Input: part model. Units: mm. Frame: model coordinates. Give positions to 0.01 mm unless a question says otherwise; leave off trailing zeros. Write each loop counter-clockwise with the first axis right and the second up, starting at its lowest first coordinate (ties: lowest second). Pieces come first, ordered by that corner, then holes. Notation, with made-up numbers: (-4.5, -4) - (7.5, -4) arc R15 cw to (7.5, 23) - close; hole circle Ø1 at (39, 61). An arc over 180 degrees is marked (long way). Use a Markdown table: item, result. Add a question column.
1. Section query A-A, the plane y = 24. Return loops of the section in (x, z), plus the area to 3 significant figures.
2. Material intervals for probe 1 along Y at (x, z) = (82, 1.5); probe 2 along Y at (x, z) = (57.5, 1.5); probe 3 along Y at (x, z) = (76.5, 2.25), sorted ascending.
3. Section query C-C, the plane x = 135.5. Return loops of the section in (y, z), plus the area to 3 significant figures.
4. Section query B-B, the plane x = 54. Return loops of the section in (y, z), plus the area to 3 significant figures.
5. Pin query (flat end, axial travel): pin 1 (0.9 mm diameter, centred on x = 24.5, y = 2, fed in from +Z); pin 2 (1.3 mm diameter, centred on x = 52.5, y = 14, fed in from +Z); pin 3 (2 mm diameter, centred on y = 10, z = 0, fed in from -X); pin 4 (10 mm diameter, centred on x = 81.5, y = 11.5, fed in from -Z). Return the tip coordinate at first contact, or that it passes through.
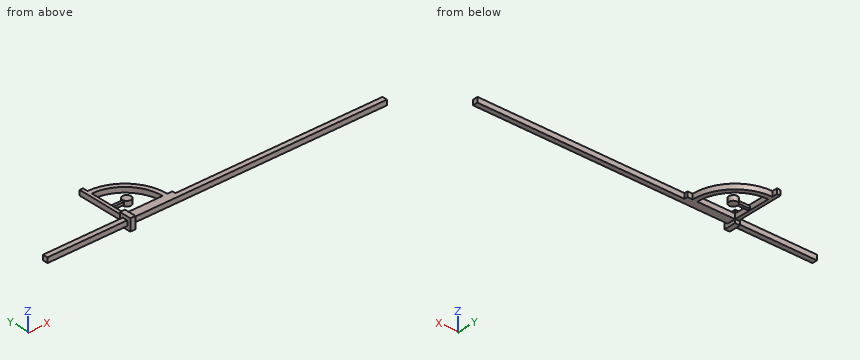
Autodesk Inventor part; units mm, degrees
ref_plane "YZ Plane" through (0, 0, 0) normal (1, 0, 0) x (0, 1, 0)
ref_plane "XZ Plane" through (0, 0, 0) normal (0, 1, 0) x (-1, 0, 0)
ref_plane "XY Plane" through (0, 0, 0) normal (0, 0, 1) x (1, 0, 0)
sketch "Skizze4" plane through (0, 0, 0) normal (0, 0, 1) x (1, 0, 0)
  line L0 (0, 0) -> (200, 0)
  line L1 (200, 0) -> (200, 3)
  line L2 (200, 3) -> (0, 3)
  line L3 (0, 3) -> (0, 0)
  dimension "d12" = 200
  dimension "d13" = 3
extrude "Extrusion4" add sketch "Skizze4" along normal blind 3
sketch "Skizze5" plane through (0, 0, 3) normal (0, 0, 1) x (1, 0, 0)
  line L0 (47, 5) -> (50, 5)
  line L1 (50, 5) -> (50, -2)
  line L2 (50, -2) -> (47, -2)
  line L3 (47, -2) -> (47, 5)
  line L4 (200, 0) -> (200, 3)
  line L5 (0, 3) -> (0, 0)
  line L6 (200, 3) -> (0, 3)
  line L7 (0, 0) -> (200, 0)
  dimension "d16" = 150
  dimension "d17" = 47
  dimension "d18" = 2
  dimension "d19" = 2
extrude "Extrusion5" add sketch "Skizze5" along normal blind 2 and the other way blind 5 contours L0 L1 L6 L3 | L6 L1 L7 L3 | L7 L1 L2 L3
sketch "Skizze6" plane through (0, 0, -2) normal (0, 0, -1) x (-1, 0, 0)
  point P0 (0, 0)
sketch "Skizze7" plane through (0, 0, 0) normal (0, 0, -1) x (-1, 0, 0)
  line L0 (-200, 3) -> (-50, 3)
  line L1 (-78, 3) -> (-50, 3)
  line L2 (-50, 3) -> (-50, 5)
  line L3 (-50, 5) -> (-78, 5)
  line L4 (-78, 5) -> (-78, 3)
  line L5 (-50, 5) -> (-48, 5)
  line L6 (-48, 5) -> (-48, 33)
  line L7 (-48, 33) -> (-50, 33)
  line L8 (-50, 33) -> (-50, 5)
  line L9 (-50, -2) -> (-50, 5)
  arc A0 (-50, 30) -> (-75, 5) centre (-50, 5) ccw
  arc A1 (-50, 27.2) -> (-72.2, 5) centre (-50, 5) ccw
  line L10 (-50, 5) -> (-59.1924, 14.1924)
  line L11 (-50, 5) -> (-37, 5) construction
  circle A2 centre (-59.1924, 14.1924) radius 2.5
  line L12 (-59.1924, 14.1924) -> (-50, 14.1924)
  line L13 (-59.1924, 14.1924) -> (-50, 14.1924)
  line L14 (-50, 14.1924) -> (-50, 13.3924)
  line L15 (-50, 13.3924) -> (-59.1924, 13.3924)
  line L16 (-59.1924, 13.3924) -> (-59.1924, 14.1924)
  line L17 (-50, 14.1924) -> (-59.1924, 14.1924)
  line L18 (-59.1924, 14.1924) -> (-59.1924, 14.9924)
  line L19 (-59.1924, 14.9924) -> (-50, 14.9924)
  line L20 (-50, 14.9924) -> (-50, 14.1924)
  line L21 (-50, 30) -> (-50, 27.2)
  line L22 (-75, 5) -> (-72.2, 5)
  point P0 (0, 0)
  dimension "d24" = 2
  dimension "d25" = 2
  dimension "d26" = 50
  dimension "d27" = 2.8
  dimension "d28" = 13
  dimension "d29" = 135
  dimension "d30" = 5
  dimension "d31" = 0.8
  dimension "d32" = 0.8
  dimension "d33" = 28
  dimension "d34" = 28
extrude "Extrusion6" add sketch "Skizze7" against normal blind 3 contours L4 L3 L2 L0 | L8 L7 L6 L5 | A0 L8 A1 L3 | L15 A2 L12 L8 | A2 L19 L18 L16 L15 L10 | L10 L15 A2 | L12 A2 L19 L8 | L15 L10 L12 A2 | L15 L16 L10 | A2 L12 L18 L19
sketch "Skizze8" plane through (0, 0, 0) normal (0, 0, -1) x (-1, 0, 0)
  arc A0 (-56.8238, 14.9924) -> (-56.8238, 13.3924) centre (-59.1924, 14.1924) ccw
  circle A1 centre (-59.1924, 14.1924) radius 2.5
  line L0 (-56.8238, 13.3924) -> (-50, 13.3924)
  line L1 (-56.8238, 13.3924) -> (-50, 13.3924)
  line L2 (-50, 13.3924) -> (-50, 14.9924)
  line L3 (-56.8238, 14.9924) -> (-50, 14.9924)
  line L4 (-50, 14.9924) -> (-56.8238, 14.9924)
  point P0 (0, 0)
extrude "Extrusion7" cut sketch "Skizze8" against normal blind 0.75 contours L3 L2 L0 A1
sketch "Skizze9" plane through (0, 0, 3) normal (0, 0, 1) x (1, 0, 0)
  arc A0 (56.8238, 13.3924) -> (56.8238, 14.9924) centre (59.1924, 14.1924) ccw
  circle A1 centre (59.1924, 14.1924) radius 2.5
  line L0 (50, 14.9924) -> (50, 27.2)
  line L1 (56.8238, 14.9924) -> (50, 14.9924)
  line L2 (50, 14.9924) -> (50, 13.3924)
  line L3 (50, 14.9924) -> (50, 13.3924)
  line L4 (50, 13.3924) -> (56.8238, 13.3924)
  point P0 (0, 0)
extrude "Extrusion8" cut sketch "Skizze9" against normal blind 0.75 contours L4 L2 L1 A1
properties part number "MiddleStick"
Result sheet:
| question | item | result |
|---|---|---|
| 1 | outline | (48, 0) - (50, 0) - (50, 3) - (48, 3) - close; (61.48, 0) - (66.25, 0) - (66.25, 3) - (61.48, 3) - close |
| 1 | area | 20.3 mm² |
| 2 | probe 1 | y = 0 to 3 |
| 2 | probe 2 | y = 0 to 5, 12.35 to 16.03, 25.89 to 28.85 |
| 2 | probe 3 | y = 0 to 5 |
| 3 | outline | (0, 0) - (3, 0) - (3, 3) - (0, 3) - close |
| 3 | area | 9.00 mm² |
| 4 | outline | (0, 0) - (5, 0) - (5, 3) - (0, 3) - close; (13.39, 0.75) - (14.99, 0.75) - (14.99, 2.25) - (13.39, 2.25) - close; (26.84, 0) - (29.68, 0) - (29.68, 3) - (26.84, 3) - close |
| 4 | area | 25.9 mm² |
| 5 | pin 1 | stops at z = 3 |
| 5 | pin 2 | stops at z = 2.25 |
| 5 | pin 3 | stops at x = 48 |
| 5 | pin 4 | passes through |
